Autodesk Inventor part; units mm, degrees
ref_plane "YZ Plane" through (0, 0, 0) normal (1, 0, 0) x (0, 1, 0)
ref_plane "XZ Plane" through (0, 0, 0) normal (0, 1, 0) x (-1, 0, 0)
ref_plane "XY Plane" through (0, 0, 0) normal (0, 0, 1) x (1, 0, 0)
sketch "Sketch1" plane through (0, 0, 0) normal (0, 1, 0) x (-1, 0, 0)
  line L0 (-63.7289, -30.1) -> (-63.7289, 0)
  circle A0 centre (-78.6786, -6.05) radius 1.05
  circle A1 centre (-76.6786, -24.05) radius 1.05
  circle A2 centre (-69.1786, -24.05) radius 1.05
  circle A3 centre (-69.1786, -6.05) radius 1.05
  circle A4 centre (-43.1593, -6.9) radius 1.05
  circle A5 centre (-44.1593, -20.12) radius 1.05
  circle A6 centre (-51.1593, -27.42) radius 1.05
  circle A7 centre (-58.1593, -20.12) radius 1.05
  circle A8 centre (-59.1593, -6.9) radius 1.05
  arc A9 (-40.0893, -1) -> (-41.0893, 0) centre (-41.0893, -1) ccw
  line L1 (-40.0893, -29.1) -> (-40.0893, -1)
  arc A10 (-41.0893, -30.1) -> (-40.0893, -29.1) centre (-41.0893, -29.1) ccw
  arc A11 (-80.8355, 0) -> (-76.7307, -30.1) centre (-42.1186, -10.05) ccw
  line L2 (-57.7093, 0) -> (-80.8355, 0)
  line L3 (-76.7307, -30.1) -> (-41.0893, -30.1)
  arc A12 (-57.7093, 0) -> (-44.6093, 0) centre (-51.1593, 0) ccw
  line L4 (-41.0893, 0) -> (-44.6093, 0)
  line L5 (-63.2793, -30.1) -> (-63.2793, 0)
  line L6 (-64.1786, 0) -> (-64.1786, -30.1)
extrude "Extrusion1" add sketch "Sketch1" against normal blind 1.5
properties part number "axis_2_bottom_L_frame(top)"
For this review, take the finished solid that the model builds, in its own axes (mm). Round coordinates to 2 decimals unless told otherwise and drop trailing zeros. Write each loop counter-clockwise with the first axis right and the second up, starting at its lowest first coordinate (ties: lowest second). Pieces come first, ordered by that corner, then holes. Notation, with made-up numbers: (-30, -25) - (14, -25) arc R23 ccw to (14, 14) - close; hole circle Ø9 at (37, 82). An arc over 180 degrees is marked (long way). Answer as CSV lines item,"result". Start each with the question number.
(1) For line 1 (X direction, y = -0.7, z = -24.5); line 2 (Z direction, x = 58.5, y = -1.3); line 3 (X direction, y = -0.05, z = -27), list the stretches that pass through material, from the lowest coordinate up.
(2) For pin 1 (1.9 mm diameter, centred on x = 69.18, z = -24.05, fed in from -Y), flat-tipped, find the tip position at first contact; note if it passes through.
(3) Add section D-D, the plane z = -27.42. State the section outline as (x, y) points.
(4) Add section C-C, the plane x = 69. State the section outline as (y, z) points, plus the area to 3 significant figures.
(5) Add section A-A, the plane y = -1.25. State how many separate pieces and enclosed holes the cut face has, plus the area to 3 significant figures.
(6) Add section B-B, the plane z = -20.12. State the section outline as (x, y) points, plus the area to 3 significant figures.
(7) Mouldability with a two-part tool opening along X and no side actions: class faces 1 (the cylindrical face through (51.3, -0.74, -6.55)), 2 (the cylindrical face through (81.78, -0.74, -15.24)), 3 (the flat face through (59, -1, -30.1)) as +X half, -X half, draft (parallel to the pull), parting line (faces both ways), or undercut.
From the geometry:
1,line 1,"x = 40.09 to 68.23, 70.13 to 75.73, 77.63 to 79.42"
1,line 2,"z = -30.1 to -21.11, -19.13 to -7.72, -6.08 to 0"
1,line 3,"x = 40.09 to 50.2, 52.12 to 78.35"
2,pin 1,"passes through"
3,outline,"(40.09, -1.5) - (50.11, -1.5) - (50.11, 0) - (40.09, 0) - close; (52.21, -1.5) - (78.15, -1.5) - (78.15, 0) - (52.21, 0) - close"
4,outline,"(-1.5, -30.1) - (0, -30.1) - (0, -25.08) - (-1.5, -25.08) - close; (-1.5, -23.02) - (0, -23.02) - (0, -7.08) - (-1.5, -7.08) - close; (-1.5, -5.02) - (0, -5.02) - (0, 0) - (-1.5, 0) - close"
4,area,"38.9 mm²"
5,separate pieces,"1"
5,enclosed holes,"9"
5,area,"1,130 mm²"
6,outline,"(40.09, -1.5) - (43.11, -1.5) - (43.11, 0) - (40.09, 0) - close; (45.21, -1.5) - (57.11, -1.5) - (57.11, 0) - (45.21, 0) - close; (59.21, -1.5) - (80.83, -1.5) - (80.83, 0) - (59.21, 0) - close"
6,area,"54.8 mm²"
7,face 1,"undercut"
7,face 2,"+X half"
7,face 3,"draft"
